Build history of the part. All positions in model axes, mm. A direction names the side the tool comes from. Round coordinates to 2 decimals unless told otherwise and drop trailing zeros. Write each loop counter-clockwise with the first axis right and the second up, starting at its lowest first coordinate (ties: lowest second). Pieces come first, ordered by that corner, then holes.
from build123d import *

# Parameters (mm, degrees)
F0_R     = 15
F1_DEPTH = 15
F2_R     = 18.5
F3_DEPTH = 64
F4_R     = 15
F5_DEPTH = 39
F6_R     = 14
F7_DEPTH = 59


with BuildPart() as f1:
    # F0 (on Front) → F1 (new body)
    with BuildSketch(Plane.XZ):
        Circle(F0_R)
    extrude(amount=F1_DEPTH)

    # F2 (on Front) → F3 (join)
    with BuildSketch(Plane.XZ):
        Circle(F2_R)
    extrude(amount=-F3_DEPTH)

    # F4 (on face) → F5 (join)
    with BuildSketch(Plane(origin=(0, 64, 0), x_dir=(-1, 0, 0), z_dir=(0, 1, 0))):
        Circle(F4_R)
    extrude(amount=F5_DEPTH)

    # F6 (on face) → F7 (join)
    with BuildSketch(Plane(origin=(0, 103, 0), x_dir=(-1, 0, 0), z_dir=(0, 1, 0))):
        Circle(F6_R)
    extrude(amount=F7_DEPTH)


solid = f1.part
1) Slice it at B-B (x = 0). Write the cut outline in (y, z), plus the area to 3 significant figures.
Results:
outline: (-15, -15) - (0, -15) - (0, -18.5) - (64, -18.5) - (64, -15) - (103, -15) - (103, -14) - (162, -14) - (162, 14) - (103, 14) - (103, 15) - (64, 15) - (64, 18.5) - (0, 18.5) - (0, 15) - (-15, 15) - close
area: 5,640 mm2
2) Wall check: L1, parallel to Y at x = -12, z = -7.5; L2, parallel to Z at x = -0.5, y = 24.5; L3, parallel to Z at x = 1, y = 107. Give the ranges that are in metal, low to high.
Results:
L1: y = -15 to 103
L2: z = -18.49 to 18.49
L3: z = -13.96 to 13.96
3) Pin check, flat tips, straight feed: pin 1 Ø2 at (x, y) = (-13.5, 113.5) entering from +Z; pin 2 Ø6 at (x, y) = (-12, 47.5) entering from -Z; pin 3 Ø6 at (y, z) = (139.5, -11.5) entering from +X; pin 4 Ø12 at (x, z) = (7, 12.5) entering from +Y. Stop position of each tip, or through.
Results:
pin 1: stops at z = 6.3
pin 2: stops at z = -16.16
pin 3: stops at x = 11.12
pin 4: stops at y = 162
4) Slice it at A-A (z = 0). Write the cut outline in (x, y).
Results:
outline: (-18.5, 0) - (-15, 0) - (-15, -15) - (15, -15) - (15, 0) - (18.5, 0) - (18.5, 64) - (15, 64) - (15, 103) - (14, 103) - (14, 162) - (-14, 162) - (-14, 103) - (-15, 103) - (-15, 64) - (-18.5, 64) - close
5) Slice it at C-C (y = 28). Write the cut outline in (x, z).
Results:
outline: circle Ø37 at (0, 0)
6) Slice it at D-D (y = 100). Write the cut outline in (x, z), plus the area to 3 significant figures.
Results:
outline: circle Ø30 at (0, 0)
area: 707 mm2
7) Which spindle directions (+Z, -Z, +X, -X, +Y, -Y) get a long thin tool onto all of the face, cutting with end or side? Do faces 1 (the flat face through (0, -15, 0)), 2 (the flat face through (-0.1, 64, 15.2)), 3 (the cylindrical face through (-14.985, -7.395, 0.66)). Say none if no direction does.
Results:
face 1: +Z, -Z, +X, -X, -Y
face 2: +Y
face 3: -Y
